The model under review builds one solid part; all positions refer to its coordinate system, in mm. A direction names the side the tool comes from. Give positions to 0.01 mm unless a question says otherwise; leave off trailing zeros. Order: outer loops, then holes, each group sorted by start corner. A loop starts at its lowest first (then second) coordinate and runs counter-clockwise, first axis right, second up.
```python
from build123d import *

# Parameters (mm, degrees)
F1_DEPTH     = 12.7
F0_W         = 25.4
F0_H         = 6.35
F2_DEPTH     = 3.175
F3_SIZE      = 7.62
F4_R         = 18.3677824361
F5_DEPTH     = 10.16
F6_W         = 8.6341705173
F6_H         = 22.7366536856
F6_W_2       = 7.7707553282
F7_DEPTH     = 12.7
F8_R         = 5.08
F9_R         = 1.736345134
F10_DEPTH    = 177.8
F11_T1_DEPTH = 31.75
F12_W        = 3.81
F12_H        = 3.810003606
F12_H_2      = 3.81
F13_DEPTH    = 25.4


# Not quite as in the source:
# - a fillet or chamfer that OpenCascade refuses, or shapes differently, is made with other operations: its cross-section is extruded or revolved along the edge and cut away or added


with BuildPart() as f1:
    # F0 (on Front) → F1 (new body, symmetric)
    with BuildSketch(Plane.XZ):
        Polygon((1.495771724, 35.256898239), (-23.904228276, 35.256898239), (-23.904228276, 27.4009877652), (-23.904228276, 21.0509877652), (-23.904228276, 9.856898239), (1.495771724, 9.856898239), align=None)
    extrude(amount=F1_DEPTH, both=True)

    # F0 (on Front) → F2 (join, symmetric)
    with BuildSketch(Plane.XZ):
        with Locations((-36.604228276, 24.2259877652)):
            Rectangle(F0_W, F0_H)
    extrude(amount=F2_DEPTH, both=True)

    # F3
    f3_edges = [f1.edges().sort_by_distance(p)[0] for p in [
        (-23.904228, 0, 35.256898),
    ]]
    chamfer(f3_edges, length=F3_SIZE)

    # F4 (on Top) → F5 (join)
    with BuildSketch(Plane.XY):
        with Locations((-12.0878415182, 0)):
            Circle(F4_R)
    extrude(amount=F5_DEPTH)

    # F6 (on Right) → F7 (join)
    with BuildSketch(Plane.YZ):
        with Locations((-8.9219780639, -11.3683268428)):
            Rectangle(F6_W, F6_H)
        with Locations((8.7780752219, -11.3683268428)):
            Rectangle(F6_W_2, F6_H)
    extrude(amount=-F7_DEPTH)

    # F8
    f8_edges = [f1.edges().sort_by_distance(p)[0] for p in [
        (-12.7, 8.778075, -22.736654),
        (-12.7, -8.921978, -22.736654),
        (0, -8.921978, -22.736654),
        (0, 8.778075, -22.736654),
    ]]
    fillet(f8_edges, radius=F8_R)

    # F9 (on Right) → F10 (cut)
    with BuildSketch(Plane.YZ):
        with Locations((0, 24.2223944515)):
            Circle(F9_R)
    extrude(amount=-F10_DEPTH, mode=Mode.SUBTRACT)

    # F11: fillet of radius 5.08 on 2 edges, made by hand

    # F11_s2 → F11_t1 (cut)
    with BuildSketch(Plane.XY.offset(8.3509877652)):
        with BuildLine():
            ThreePointArc((-44.224228276, 3.175), (-47.8163307244, 1.6871024484), (-49.304228276, -1.905))
            Line((-49.304228276, -1.905), (-49.304228276, 3.175))
            Line((-49.304228276, 3.175), (-44.224228276, 3.175))
        make_face()
        with BuildLine():
            ThreePointArc((-44.224228276, -3.175), (-47.8163307244, -1.6871024484), (-49.304228276, 1.905))
            Line((-49.304228276, 1.905), (-49.304228276, -3.175))
            Line((-49.304228276, -3.175), (-44.224228276, -3.175))
        make_face()
    extrude(amount=F11_T1_DEPTH, mode=Mode.SUBTRACT)

    # F12 (on Right) → F13 (cut)
    with BuildSketch(Plane.YZ):
        with Locations((7.1409824217, 30.2377566695)):
            Rectangle(F12_W, F12_H)
        with Locations((-8.4303260025, 30.2377548665)):
            Rectangle(F12_W, F12_H_2)
    extrude(amount=-F13_DEPTH, mode=Mode.SUBTRACT)


solid = f1.part
```
Item 1: For line 1 (Z direction, x = -37, y = 0); line 2 (Y direction, x = -8, z = -15); line 3 (Z direction, x = -14, y = 0), list the stretches that pass through material, from the lowest coordinate up.
Values found:
line 1: z = 21.05 to 22.49, 25.96 to 27.4
line 2: y = -13.24 to -4.6, 4.89 to 12.66
line 3: z = 0 to 22.49, 25.96 to 35.26
Item 2: For faces 5 (the cylindrical face through (-11.25, 8.83, -21.21)), 6 (the flat face through (0, 9, -9)), 7 (the flat face through (-6, -4.605, -12)), 8 (the flat face through (-20.15, 0.18, 31.39)), 9 (the flat face through (-24.1, -1.3, 10.16)), list the 3-axis set-ups (+Z, -Z, +X, -X, +Y, -Y) from which the entire face can be reached by the end or side of a thin tool; tool diameter is ignored.
Values found:
face 5: -Z, -X, +Y, -Y
face 6: -Z, +X, +Y, -Y
face 7: -Z, +X, -X
face 8: +Z, -X, +Y, -Y
face 9: -X
Item 3: Take a section at B-B (z = 16). Give the boundary of the cut face in (x, y), and give its area (3 significant figures).
Values found:
outline: (-23.9, -12.7) - (1.5, -12.7) - (1.5, 12.7) - (-23.9, 12.7) - close
area: 645 mm2
Item 4: Take a section at A-A (x = -22). Give the boundary of the cut face in (y, z).
Values found:
outline: (-15.46, 0) - (15.46, 0) - (15.46, 10.16) - (12.7, 10.16) - (12.7, 29.54) - (9.05, 29.54) - (9.05, 28.33) - (5.24, 28.33) - (5.24, 29.54) - (-6.53, 29.54) - (-6.53, 28.33) - (-10.34, 28.33) - (-10.34, 29.54) - (-12.7, 29.54) - (-12.7, 10.16) - (-15.46, 10.16) - close; hole circle Ø3.47 at (0, 24.22)
Item 5: Take a section at C-C (x = -32.5). Give the boundary of the cut face in (y, z) (3 decimals), and give its area (3 significant figures).
Values found:
outline: (-3.175, 21.051) - (3.175, 21.051) - (3.175, 27.401) - (-3.175, 27.401) - close; hole circle Ø3.473 at (0, 24.222)
area: 30.9 mm2
Item 6: Draft analysis for pull direction Y (two halves, no side actions). For faces 1 (the flat face through (-6, -13.239, -12)), 2 (the flat face through (-12.7, 9, -9)), 3 (the flat face through (-34, 3.175, 24)), 4 (the flat face through (0, 7, 30)), state which applies: released by +Y, released by -Y, zero draft, split by the parting line, or undercut.
Values found:
face 1: released by -Y
face 2: zero draft
face 3: released by +Y
face 4: undercut
Item 7: Take a section at D-D (z = 7). Give the boundary of the cut face in (x, y), and give its area (3 significant figures).
Values found:
outline: circle Ø36.74 at (-12.09, 0)
area: 1,060 mm2
Item 8: Clearance check with flat-ended pins moving along their axes: pin 1 Ø12 at (x, z) = (-21, 19) entering from -Y; pin 2 Ø2 at (x, y) = (-23, 11) entering from +Z; pin 3 Ø10 at (y, z) = (-5, 3) entering from -X; pin 4 Ø4 at (y, z) = (-2.5, -17) entering from -X. State where each tip first meets the part, or that it passes through.
Values found:
pin 1: stops at y = -12.7
pin 2: stops at z = 29.54
pin 3: stops at x = -30.46
pin 4: passes through
